from build123d import *

# Parameters (mm, degrees)
F1_DEPTH = 5.715
F2_R     = 1.651
F3_DEPTH = 3.811
F2_R_2   = 2.794
F4_DEPTH = 1.524


with BuildPart() as f1:
    # F0 (on Front) → F1 (new body, symmetric)
    with BuildSketch(Plane.XZ):
        Polygon((-19.7866, 3.81), (-19.7866, 0), (-4.5466, 0), (-4.5466, 9.0932), (4.5466, 9.0932), (4.5466, 0), (19.7866, 0), (19.7866, 3.81), (8.3566, 3.81), (8.3566, 12.9032), (-8.3566, 12.9032), (-8.3566, 3.81), align=None)
    extrude(amount=F1_DEPTH, both=True)

    # F2 (on face) → F3 (cut, through all)
    with BuildSketch(Plane.XY.offset(3.81)):
        with Locations((-13.97, 0)):
            Circle(F2_R)
        with Locations((13.97, 0)):
            Circle(F2_R)
    extrude(amount=-F3_DEPTH, mode=Mode.SUBTRACT)

    # F2 (on face) → F4 (cut)
    with BuildSketch(Plane.XY.offset(3.81)):
        with Locations((13.97, 0)):
            Circle(F2_R_2)
        with Locations((13.97, 0)):
            Circle(F2_R, mode=Mode.SUBTRACT)
        with Locations((-13.97, 0)):
            Circle(F2_R_2)
        with Locations((-13.97, 0)):
            Circle(F2_R, mode=Mode.SUBTRACT)
    extrude(amount=-F4_DEPTH, mode=Mode.SUBTRACT)


solid = f1.part
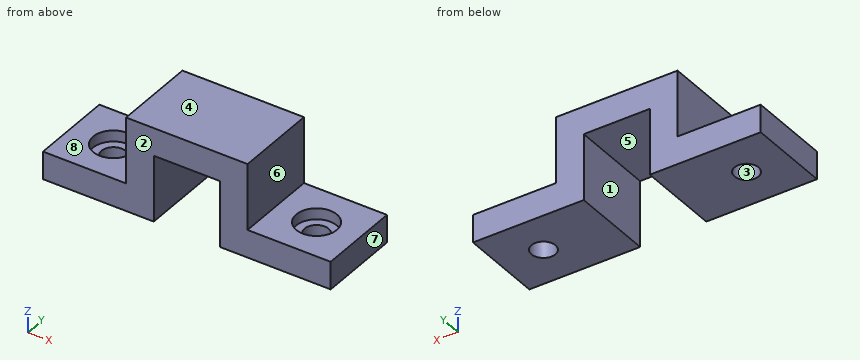
Read the model definition and answer for the solid it produces. Units are mm, in the model's axes. Face numbers are marked on the shaded views. A direction names the side the tool comes from. Give positions to 0.01 mm unless a question says otherwise; leave off trailing zeros. Loops run counter-clockwise (first coordinate to the right, second up) from the corner with the lowest first, then second, coordinate; pieces in that order, holes last. Notation, with made-up numbers: M -34,9.5 L 1,9.5 A10 cw 1,21.5 Z; hole C 78.5,12 d10. An arc over 180 degrees is marked long. Write each question's results on one line, items separated by ' | '.
1. Section C-C on x = 13.97 is taken. Give the vertices of the cut face in (y, z) (3 decimals).
Values:
outline: M -5.715,0 L -1.651,0 L -1.651,2.286 L -2.794,2.286 L -2.794,3.81 L -5.715,3.81 Z; M 1.651,0 L 5.715,0 L 5.715,3.81 L 2.794,3.81 L 2.794,2.286 L 1.651,2.286 Z
2. The mould has two halves that part along Y. Classify the marked faces 1, 2 and 3: pulls with the +Y half, pulls with the -Y half, needs draft (parallel to the pull), parting line crosses it, or undercut.
Values:
face 1: needs draft | face 2: pulls with the -Y half | face 3: undercut
3. Straight lines are drawn through the part: line 1 (Y direction, x = -13.97, z = 3.1) (3 decimals); line 2 (X direction, y = 4.5, z = 7.25); line 3 (X direction, y = 0.75, z = 3.5). For each, find the intervals that lie inside material, in ascending order. Write a range as [from, to].
Values:
line 1: y = [-5.715, -2.794], [2.794, 5.715] | line 2: x = [-8.36, -4.55], [4.55, 8.36] | line 3: x = [-19.79, -16.66], [-11.28, -4.55], [4.55, 11.28], [16.66, 19.79]
4. Section D-D on x = -2.5 is taken. Give the vertices of the cut face in (y, z) (3 decimals).
Values:
outline: M -5.715,9.093 L 5.715,9.093 L 5.715,12.903 L -5.715,12.903 Z
5. Section B-B on z = 7.5 is taken. Give the vertices of the cut face in (x, y) (3 decimals), plus the area to 3 significant figures.
Values:
outline: M -8.357,-5.715 L -4.547,-5.715 L -4.547,5.715 L -8.357,5.715 Z; M 4.547,-5.715 L 8.357,-5.715 L 8.357,5.715 L 4.547,5.715 Z | area: 87.1 mm^2
6. Section A-A on y = 0 is taken. Give the vertices of the cut face in (x, z), plus the area to 3 significant figures.
Values:
outline: M -19.79,0 L -15.62,0 L -15.62,2.29 L -16.76,2.29 L -16.76,3.81 L -19.79,3.81 Z; M -12.32,0 L -4.55,0 L -4.55,9.09 L 4.55,9.09 L 4.55,0 L 12.32,0 L 12.32,2.29 L 11.18,2.29 L 11.18,3.81 L 8.36,3.81 L 8.36,12.9 L -8.36,12.9 L -8.36,3.81 L -11.18,3.81 L -11.18,2.29 L -12.32,2.29 Z; M 15.62,0 L 19.79,0 L 19.79,3.81 L 16.76,3.81 L 16.76,2.29 L 15.62,2.29 Z | area: 188 mm^2
7. Given pin 1 (2.5 mm diameter, centred on y = 0.5, z = 8.5, fed in from +X); pin 2 (5 mm diameter, centred on x = 13.97, y = 0, fed in from +Z); pin 3 (6 mm diameter, centred on y = -1.5, z = 8, fed in from -X), each flat-ended and moving along its own axis, determine where each tip first touches the part or whether it passes through.
Values:
pin 1: stops at x = 8.36 | pin 2: stops at z = 2.29 | pin 3: stops at x = -8.36
8. A tool of negligible diameter and unlimited length cuts with its end or side. For the marked faces 4, 5, 6, 7 and 8, from which of +Z, -Z, +X, -X, +Y, -Y can it reach the whole face along a straight path? Write none if from no direction.
Values:
face 4: +Z, +X, -X, +Y, -Y | face 5: -Z, +Y, -Y | face 6: +Z, +X, +Y, -Y | face 7: +Z, -Z, +X, +Y, -Y | face 8: +Z, -X, +Y, -Y
